Autodesk Inventor part; units mm, degrees
ref_plane "YZ Plane" through (0, 0, 0) normal (1, 0, 0) x (0, 1, 0)
ref_plane "XZ Plane" through (0, 0, 0) normal (0, 1, 0) x (-1, 0, 0)
ref_plane "XY Plane" through (0, 0, 0) normal (0, 0, 1) x (1, 0, 0)
sketch "Sketch1" plane through (0, 0, 0) normal (0, 1, 0) x (-1, 0, 0)
  circle A0 centre (0, 0) radius 9.5 construction
  circle A1 centre (0, 0) radius 9.5 construction
  line L0 (0, 0) -> (9.5, 0) construction
  line L1 (0, 0) -> (6.7175, -6.7175) construction
  circle A2 centre (6.7175, -6.7175) radius 1.375
  line L2 (0, 0) -> (6.7175, 6.7175) construction
  circle A3 centre (6.7175, 6.7175) radius 1.375
  circle A4 centre (-6.7175, -6.7175) radius 1.375
  circle A5 centre (-6.7175, 6.7175) radius 1.375
  circle A6 centre (0, 0) radius 4
  line L3 (-6.7175, -6.7175) -> (6.7175, 6.7175) construction
  arc A7 (-8.4853, -4.9497) -> (-4.9497, -8.4853) centre (-6.7175, -6.7175) ccw
  arc A8 (8.4853, 4.9497) -> (4.9497, 8.4853) centre (6.7175, 6.7175) ccw
  line L4 (-6.7175, 6.7175) -> (6.7175, -6.7175) construction
  arc A9 (-4.9497, 8.4853) -> (-8.4853, 4.9497) centre (-6.7175, 6.7175) ccw
  arc A10 (4.9497, -8.4853) -> (8.4853, -4.9497) centre (6.7175, -6.7175) ccw
  line L5 (4.7625, -2.7496) -> (0, -5.4993)
  line L6 (0, -5.4993) -> (-4.7625, -2.7496)
  line L7 (-4.7625, -2.7496) -> (-4.7625, 2.7496)
  line L8 (-4.7625, 2.7496) -> (0, 5.4993)
  line L9 (0, 5.4993) -> (4.7625, 2.7496)
  line L10 (4.7625, 2.7496) -> (4.7625, -2.7496)
  line L11 (-4.9497, -8.4853) -> (-1.245, -4.7805)
  line L12 (4.7625, 1.227) -> (8.4853, 4.9497)
  line L13 (4.9497, 8.4853) -> (1.245, 4.7805)
  line L14 (-4.7625, -1.227) -> (-8.4853, -4.9497)
  line L15 (-8.4853, 4.9497) -> (-4.7625, 1.227)
  line L16 (1.245, -4.7805) -> (4.9497, -8.4853)
  line L17 (8.4853, -4.9497) -> (4.7625, -1.227)
  line L18 (-1.245, 4.7805) -> (-4.9497, 8.4853)
  circle A11 centre (0, 0) radius 4.5
  circle A12 centre (0, 0) radius 6.35
  point P0 (4.7625, 0)
  point P1 (-2.3597, -5.8953)
  point P2 (2.3597, -5.8953)
  point P3 (-5.8953, 2.3597)
  point P4 (-5.8953, -2.3597)
  point P5 (2.3597, 5.8953)
  point P6 (-2.3597, 5.8953)
  point P7 (5.8953, 2.3597)
  point P8 (5.8953, -2.3597)
  dimension "d1" = 19
  dimension "d0" = 19
  dimension "d2" = 2.75
  dimension "d3" = 45
  dimension "d4" = 2.75
  dimension "d7" = 360
  dimension "d9" = 8
  dimension "d10" = 5
  dimension "d11" = 5
  dimension "d13" = 9.525
  dimension "d16" = 9
  dimension "d22" = 12.7
extrude "Extrusion1" add sketch "Sketch1" along normal blind 3 contours L14 A12 L11 A7 | A12 L15 L7 L14 | L14 L7 L6 L11 A12 | L11 L6 L5 L16 A12 | L7 L8 L9 L10 L5 L6 | A12 L18 L8 L7 L15 | L15 A9 L18 A12 | A12 L17 A10 L16 | L16 L5 L10 L17 A12 | A12 L13 L9 L8 L18 | L17 L10 L12 A12 | A12 L12 L10 L9 L13 | L13 A8 L12 A12 | A11
extrude "Extrusion2" add sketch "Sketch1" along normal blind 5.5 contours L7 L8 L9 L10 L5 L6 | A11
extrude "Extrusion3" add sketch "Sketch1" along normal blind 10.5 contours A11
fillet "Fillet1" radius 3.175 8 edges at (2.3597, 1.5, -5.8953) (-2.3597, 1.5, -5.8953) (-5.8953, 1.5, 2.3597) (-5.8953, 1.5, -2.3597) (-2.3597, 1.5, 5.8953) (2.3597, 1.5, 5.8953) (5.8953, 1.5, -2.3597) (5.8953, 1.5, 2.3597)
equation "\"d1\" = d0"
equation "\"d2\" = d4"
properties part number "Custom Base" material "Aluminum 6061"
Read the model definition and answer for the solid it produces. Units are mm, in the model's axes. A direction names the side the tool comes from. Give positions to 0.01 mm unless a question says otherwise; leave off trailing zeros. Loops run counter-clockwise (first coordinate to the right, second up) from the corner with the lowest first, then second, coordinate; pieces in that order, holes last. Notation, with made-up numbers: (0, 26) -> (34, 26) arc R15 cw to (34, 32) -> close; hole circle Ø8 at (16, 21). An arc over 180 degrees is marked (long way). Answer as CSV lines item,"result".
Item 1: Find section D-D on z = 7.75. Give the vertices of the cut face in (x, y).
Returned:
outline,"(-8.99, 0) -> (-7.63, 0) -> (-7.63, 3) -> (-8.99, 3) -> close; (-5.81, 0) -> (-4.21, 0) -> (-4.21, 3) -> (-5.81, 3) -> close; (4.21, 0) -> (5.81, 0) -> (5.81, 3) -> (4.21, 3) -> close; (7.63, 0) -> (8.99, 0) -> (8.99, 3) -> (7.63, 3) -> close"
Item 2: Find section C-C on y = 4. Give the vertices of the cut face in (x, z).
Returned:
outline,"(-4.76, -2.75) -> (0, -5.5) -> (4.76, -2.75) -> (4.76, 2.75) -> (0, 5.5) -> (-4.76, 2.75) -> close; hole circle Ø8 at (0, 0)"
Item 3: Determine the mould class of faces 1 (the face through (-2.41, 4.23, -4.11)), 2 (the face through (0.867, 5.176, 3.905)), 3 (the face through (4, 3, -4)) for opening direction X: +X half, -X half, draft (parallel to the pull), parting line (faces both ways), or undercut.
Returned:
face 1,"-X half"
face 2,"undercut"
face 3,"draft"
Item 4: Consider line 1 (Y direction, x = 3.25, z = -4); line 2 (Z direction, x = 3.25, y = 6.5); line 3 (X direction, y = 1, z = -2.5). Determine where each line is inside the solid, lowest interval first. Write a range as [from, to].
Returned:
line 1,"y = [0, 3]"
line 2,"z = [-3.11, -2.33], [2.33, 3.11]"
line 3,"x = [-6.45, -3.12], [3.12, 6.45]"
Item 5: Find section B-B on x = 5.75. Give the vertices of the cut face in (y, z), plus the area to 3 significant figures.
Returned:
outline,"(0, -9.02) -> (3, -9.02) -> (3, -7.69) -> (0, -7.69) -> close; (0, -5.74) -> (3, -5.74) -> (3, 5.74) -> (0, 5.74) -> close; (0, 7.69) -> (3, 7.69) -> (3, 9.02) -> (0, 9.02) -> close"
area,"42.4 mm²"
Item 6: For faces 4 (the face through (4.762, 4, 0)), 5 (the face through (-4.762, 4, 0)), 6 (the face through (4.286, 1.479, 7.822)), determine the directions among +Z, -Z, +X, -X, +Y, -Y from which every point of the face is accessible in a straight line to the end or side of a thin tool.
Returned:
face 4,"+Z, -Z, +X, +Y"
face 5,"+Z, -Z, -X, +Y"
face 6,"+Z, +Y, -Y"
Item 7: Find section A-A on z = 0. Give the vertices of the cut face in (x, y).
Returned:
outline,"(-6.35, 0) -> (-4, 0) -> (-4, 10.5) -> (-4.5, 10.5) -> (-4.5, 5.5) -> (-4.76, 5.5) -> (-4.76, 3) -> (-6.35, 3) -> close; (4, 0) -> (6.35, 0) -> (6.35, 3) -> (4.76, 3) -> (4.76, 5.5) -> (4.5, 5.5) -> (4.5, 10.5) -> (4, 10.5) -> close"
Item 8: Each of these flat-tipped pins is pushed along its axis until it touches: pin 1 (1.2 mm diameter, centred on y = 4.5, z = 1, fed in from +X); pin 2 (1.5 mm diameter, centred on y = 8, z = -6.5, fed in from -X); pin 3 (0.8 mm diameter, centred on y = 4, z = 0.5, fed in from -X); pin 4 (3 mm diameter, centred on y = 7, z = -5, fed in from +X). Where does it stop, or does it pass through?
Returned:
pin 1,"stops at x = 4.76"
pin 2,"passes through"
pin 3,"stops at x = -4.76"
pin 4,"stops at x = 2.83"
